Answer from the drawing. Dimensions are ordinates in mm from the lowest x, y and z of the part. A direction names the side the tool comes from. Give positions to 0.01 mm unless a question says otherwise; leave off trailing zeros. Write each loop counter-clockwise with the first axis right and the second up, starting at its lowest first coordinate (ties: lowest second). Pieces come first, ordered by that corner, then holes. Notation, with made-up numbers: (89, 30.5) - (129, 30.5) arc R26 cw to (129, 51.5) - close; hole circle Ø6 at (41, 16.5). An arc over 180 degrees is marked (long way). Write item = value, one per line.
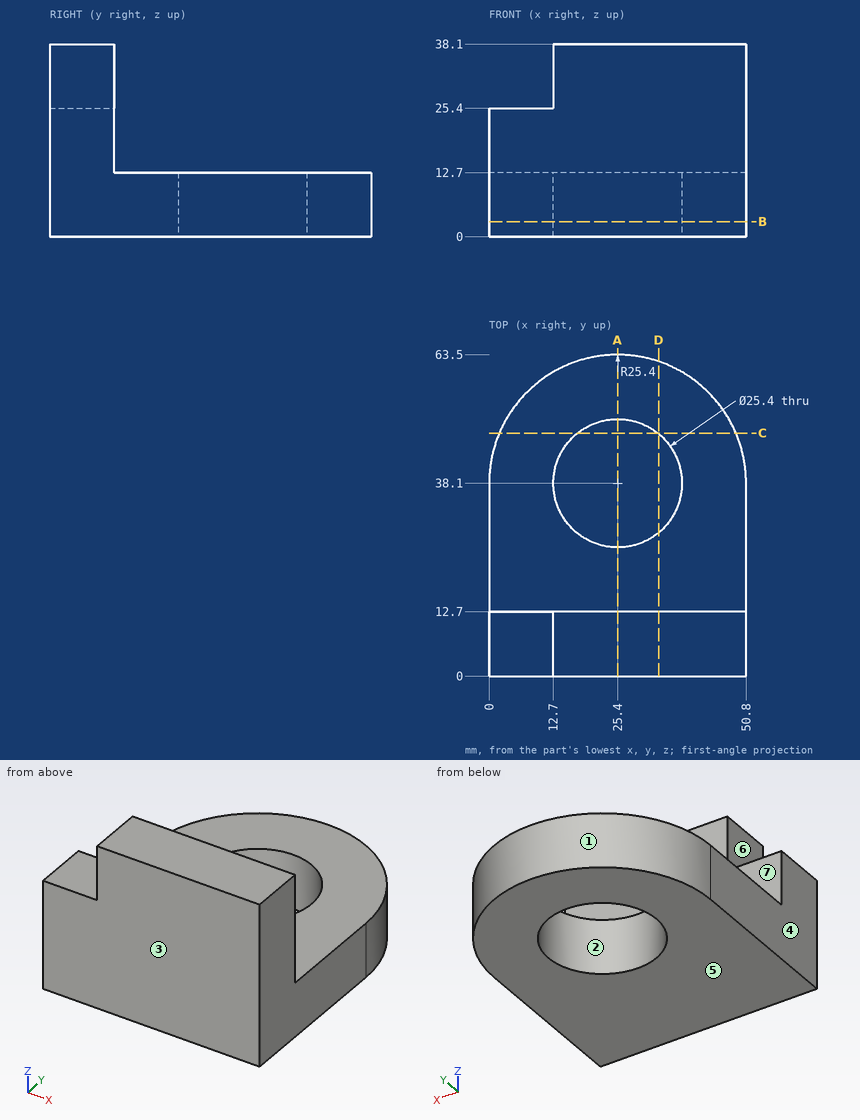
1. Given pin 1 (7.5 mm diameter, centred on x = 26, z = 29, fed in from +Y); pin 2 (10 mm diameter, centred on x = 7, y = 7.5, fed in from +Z); pin 3 (1.5 mm diameter, centred on x = 37, y = 48.5, fed in from +Z), each flat-ended and moving along its own axis, determine where each tip first touches the part or whether it passes through.
Solution:
pin_1 = 12.7
pin_2 = 25.4
pin_3 = 12.7
2. Find section B-B, the plane z = 3. Give the vertices of the cut face in (x, y), then the cut area to 3 significant figures.
Solution:
outline = (0, 0) - (50.8, 0) - (50.8, 38.1) arc R25.4 ccw to (0, 38.1) - close; hole circle Ø25.4 at (25.4, 38.1)
area = 2,440 mm^2
3. Find section C-C, the plane y = 48. Give the vertices of the cut face in (x, z).
Solution:
outline = (2.01, 0) - (17.45, 0) - (17.45, 12.7) - (2.01, 12.7) - close; (33.35, 0) - (48.79, 0) - (48.79, 12.7) - (33.35, 12.7) - close
4. A tool of negligible diameter and unlimited length cuts with its end or side. For the marked faces 5, 6 and 7, from which of +Z, -Z, +X, -X, +Y, -Y can it reach the whole face along a straight path? Write none if from no direction.
Solution:
face_5 = -Z, +X, -X, +Y, -Y
face_6 = +Z, -X, +Y, -Y
face_7 = +Z, +X, -X, +Y
5. Find section D-D, the plane x = 33.5. Give the vertices of the cut face in (y, z).
Solution:
outline = (0, 0) - (28.32, 0) - (28.32, 12.7) - (12.7, 12.7) - (12.7, 38.1) - (0, 38.1) - close; (47.88, 0) - (62.17, 0) - (62.17, 12.7) - (47.88, 12.7) - close
6. For a pull along Y with two mould halves and no side action, classify the marked faces 1, 2, 3 and 4 as pulls with the +Y half, pulls with the -Y half, needs draft (parallel to the pull), parting line crosses it, or undercut.
Solution:
face_1 = pulls with the +Y half
face_2 = undercut
face_3 = pulls with the -Y half
face_4 = needs draft
7. Find section A-A, the plane x = 25.4. Give the vertices of the cut face in (y, z).
Solution:
outline = (0, 0) - (25.4, 0) - (25.4, 12.7) - (12.7, 12.7) - (12.7, 38.1) - (0, 38.1) - close; (50.8, 0) - (63.5, 0) - (63.5, 12.7) - (50.8, 12.7) - close
8. Straight lines are drawn through the part: line 1 (Y direction, x = 25, z = 4); line 2 (X direction, y = 38, z = 5); line 3 (Z direction, x = 23, y = 16.5). For each, find the intervals that lie inside material, in ascending order.
Solution:
line_1 = 0 to 25.41, 50.79 to 63.5
line_2 = 0 to 12.7, 38.1 to 50.8
line_3 = 0 to 12.7
